Here's how the part is built. I have some questions about the finished solid (model axes, mm). Give positions to 0.01 mm unless a question says otherwise; leave off trailing zeros. Loops run counter-clockwise (first coordinate to the right, second up) from the corner with the lowest first, then second, coordinate; pieces in that order, holes last. Notation, with made-up numbers: (31, -9) -> (69, -9) arc R10 ccw to (69, 0) -> close; hole circle Ø1 at (-4.5, 47.5). An arc over 180 degrees is marked (long way). Answer in a Markdown table with one row per item. Add a question column.
Item 1: If we section it at A-A (x = 73.3): Write out the boundary of the cut face in (y, z).
Item 2: For P1, Ø2, axis at x = 69.5, y = 54.5, coming from the -Z side; P2, Ø1.9, axis at x = 7, y = 59, coming from the -Z side, each with a flat end and sliding along its axis, tell me the tip position at first contact or that it passes through.
Item 3: If I drill on line 1 (Y direction, x = 73.3, z = 1.2), over which ranges is the centre line in solid material (lowest first)?
Item 4: If we section it at B-B (y = 7): Write out the boundary of the cut face in (x, z).
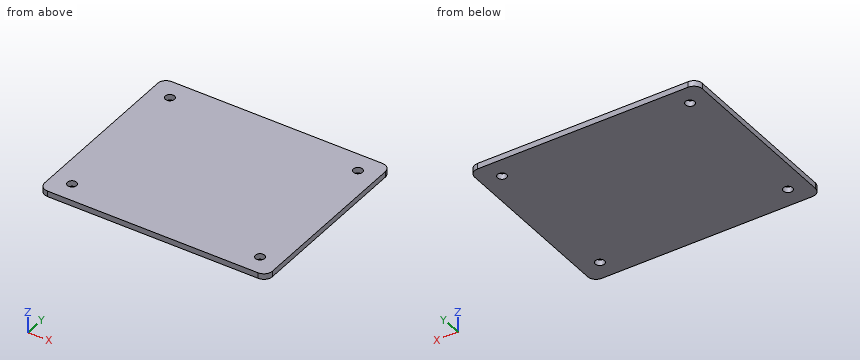
```python
from build123d import *

# Parameters (mm, degrees)
SKETCH1_W                  = 80.3
SKETCH1_H                  = 66
BOSS_EXTRUDE1_DEPTH        = 2
F_3_2_3_2_DIAMETER_HOLE1_D = 3.2
FILLET1_R                  = 3


with BuildPart() as part:
    # Sketch1 → Boss-Extrude1 (new body)
    with BuildSketch(Plane.XY):
        with Locations((40.15, 33)):
            Rectangle(SKETCH1_W, SKETCH1_H)
    extrude(amount=BOSS_EXTRUDE1_DEPTH)

    # Ø3.2 (3.2) Diameter Hole1 (through all)
    with Locations(Plane.XY.offset(2)):
        with Locations((7, 59), (73.3, 59), (73.3, 7), (7, 7)):
            Hole(F_3_2_3_2_DIAMETER_HOLE1_D / 2)

    # Fillet1
    fillet1_edges = [part.edges().sort_by_distance(p)[0] for p in [
        (0, 66, 1),
        (80.3, 66, 1),
        (80.3, 0, 1),
        (0, 0, 1),
    ]]
    fillet(fillet1_edges, radius=FILLET1_R)


solid = part.part
```
Recorded:
| question | item | result |
|---|---|---|
| 1 | outline | (0, 0) -> (5.4, 0) -> (5.4, 2) -> (0, 2) -> close; (8.6, 0) -> (57.4, 0) -> (57.4, 2) -> (8.6, 2) -> close; (60.6, 0) -> (66, 0) -> (66, 2) -> (60.6, 2) -> close |
| 2 | P1 | stops at z = 0 |
| 2 | P2 | passes through |
| 3 | line 1 | y = 0 to 5.4, 8.6 to 57.4, 60.6 to 66 |
| 4 | outline | (0, 0) -> (5.4, 0) -> (5.4, 2) -> (0, 2) -> close; (8.6, 0) -> (71.7, 0) -> (71.7, 2) -> (8.6, 2) -> close; (74.9, 0) -> (80.3, 0) -> (80.3, 2) -> (74.9, 2) -> close |
